Can you work these out from the model? Positions are in its coordinate system, mm. A direction names the side the tool comes from. Coordinates: 2 decimals unless noted, no trailing zeros. Order: outer loops, then holes, each group sorted by start corner. A loop starts at its lowest first (then second) coordinate and runs counter-clockwise, first axis right, second up. Notation, with made-up numbers: (50, -38.75) - (104, -38.75) arc R12 cw to (104, -32.75) - close; hole circle Ø10 at (-28.75, -39.75). An arc over 180 degrees is marked (long way). Use a Markdown table: item, result. Add a question column.
(1) We'd pull the mould along X, two halves only. Please class faces 1 (the flat face through (6, 3, 0)), 2 (the flat face through (0, 6, 0)), 3 (the cylindrical face through (4.6, -0.4, 0.3)): pulls with the +X half, pulls with the -X half, needs draft (parallel to the pull), parting line crosses it, or undercut.
(2) For pin 1 Ø3 at (x, y) = (-3, -4) entering from -Z; pin 2 Ø6 at (x, y) = (4, -18) entering from -Z; pin 3 Ø3 at (y, z) = (-13, -1) entering from +X; pin 4 Ø2 at (x, z) = (-2, -1) entering from -Y, each with a flat end and sliding along its axis, tell me the tip position at first contact or that it passes through.
(3) On a 3-axis mill with a long thin cutter (end or side, diameter ignored), from which of +Z, -Z, +X, -X, +Y, -Y can I reach the whole of each face in a straight line? I mean faces 4 (the cylindrical face through (-5.4, -0.4, 0.3)), 5 (the flat face through (-6, 3, 0)). Say none if no direction works.
(4) I want a section at A-A (x = 5). List the corners of the cut face in (y, z) for me.
(5) If I drill on L1, parallel to Y at x = 2.5, z = -2; L2, parallel to X at y = -9, z = -0.25; L3, parallel to Y at x = 5.75, z = -4.25, over which ranges is the centre line in solid material (lowest first)? Write a range as [from, to].
(6) I want a section at C-C (z = 4). List the corners of the cut face in (x, y) for me.
(7) I want a section at D-D (x = 0). List the corners of the cut face in (y, z) for me.
(8) I want a section at B-B (y = -13). List the corners of the cut face in (x, z) for me, and give its area (3 significant figures).
Autodesk Inventor part; units mm, degrees
ref_plane "YZ Plane" through (0, 0, 0) normal (1, 0, 0) x (0, 1, 0)
ref_plane "XZ Plane" through (0, 0, 0) normal (0, 1, 0) x (-1, 0, 0)
ref_plane "XY Plane" through (0, 0, 0) normal (0, 0, 1) x (1, 0, 0)
sketch "Эскиз7" plane through (0, 0, 0) normal (0, 1, 0) x (-1, 0, 0)
  line L0 (-6, 6) -> (6, 6)
  line L1 (6, 6) -> (6, -6)
  line L2 (6, -6) -> (-6, -6)
  line L3 (-6, -6) -> (-6, 6)
  line L4 (-6, 6) -> (6, -6) construction
  line L5 (6, 6) -> (-6, -6) construction
  point P0 (0, 0)
  dimension "d12" = 12
  dimension "d13" = 12
extrude "Выдавливание2" add sketch "Эскиз7" along normal blind 6
fillet "Сопряжение1" radius 0.5 1 edges at (6, 6, 0)
fillet "Сопряжение2" radius 0.5 13 edges at (6, 2.75, 6) (5.8536, 5.8536, 6) (-0.25, 6, 6) (-6, 0, 0) (6, 0, 0) (5.8536, 5.8536, -6) (-0.25, 6, -6) (6, 2.75, -6) (-6, 3, -6) (-6, 6, 0) (0, 0, 6) (-6, 3, 6) (0, 0, -6)
sketch "Эскиз8" plane through (0, 0, 0) normal (0, -1, 0) x (1, 0, 0)
  line L0 (0, 0) -> (-5, 0)
  line L1 (0, 0) -> (5, 0)
  circle A0 centre (-5, 0) radius 0.5
  circle A1 centre (5, 0) radius 0.5
  line L2 (5.5, -5.5) -> (5.5, 5.5)
  dimension "d18" = 5
  dimension "d19" = 5
extrude "Выдавливание3" add sketch "Эскиз8" along normal blind 1
fillet "Сопряжение3" radius 0.2 1 edges at (-5.5, -1, 0)
fillet "Сопряжение4" radius 0.2 1 edges at (4.5, -1, 0)
sketch "Эскиз10" plane through (-5, -1, 0) normal (0, -1, 0) x (1, 0, 0)
  circle A0 centre (0, 0) radius 0.3
  point P0 (5, 0)
extrude "Выдавливание4" add sketch "Эскиз10" along normal blind 24
sketch "Эскиз11" plane through (5, -1, 0) normal (0, -1, 0) x (1, 0, 0)
  circle A0 centre (0, 0) radius 0.3
  circle A1 centre (0, 0) radius 0.3
  point P0 (-5, 0)
extrude "Выдавливание5" add sketch "Эскиз11" along normal blind 24
equation "\"Радиус_гибки\" = Толщина"
equation "\"Ширина_просечки\" = Толщина"
equation "\"Глубина_просечки\" = 0.5 * Толщина"
equation "\"Размер_просечки\" = 4 * Толщина"
equation "\"Мин_остаток\" = 2 * Толщина"
equation "\"Радиус_перехода\" = Радиус_гибки"
equation "\"Радиус_Якоби\" = Радиус_гибки"
equation "\"Размер_зазора\" = Толщина"
Answers follow:
| question | item | result |
|---|---|---|
| 1 | face 1 | pulls with the +X half |
| 1 | face 2 | needs draft |
| 1 | face 3 | undercut |
| 2 | pin 1 | passes through |
| 2 | pin 2 | stops at z = -0.3 |
| 2 | pin 3 | stops at x = 5.3 |
| 2 | pin 4 | stops at y = 0 |
| 3 | face 4 | -Y |
| 3 | face 5 | +Z, -Z, -X, +Y, -Y |
| 4 | outline | (-25, -0.3) - (-1, -0.3) arc R0.2 ccw to (-0.8, -0.5) - (0, -0.5) - (0, -5.5) arc R0.5 ccw to (0.5, -6) - (5.5, -6) arc R0.5 ccw to (6, -5.5) - (6, 5.5) arc R0.5 ccw to (5.5, 6) - (0.5, 6) arc R0.5 ccw to (0, 5.5) - (0, 0.5) - (-0.8, 0.5) arc R0.2 ccw to (-1, 0.3) - (-25, 0.3) - close |
| 5 | L1 | y = [0, 6] |
| 5 | L2 | x = [-5.17, -4.83], [4.83, 5.17] |
| 5 | L3 | y = [0.07, 5.93] |
| 6 | outline | (-6, 0.5) arc R0.5 ccw to (-5.5, 0) - (5.5, 0) arc R0.5 ccw to (6, 0.5) - (6, 5.5) arc R0.5 ccw to (5.5, 6) - (-5.5, 6) arc R0.5 ccw to (-6, 5.5) - close |
| 7 | outline | (0, -5.5) arc R0.5 ccw to (0.5, -6) - (5.5, -6) arc R0.5 ccw to (6, -5.5) - (6, 5.5) arc R0.5 ccw to (5.5, 6) - (0.5, 6) arc R0.5 ccw to (0, 5.5) - close |
| 8 | outline | circle Ø0.6 at (-5, 0); circle Ø0.6 at (5, 0) |
| 8 | area | 0.565 mm² |
